Model file for the job. Use its own axes, mm. A direction names the side the tool comes from. Coordinates: 2 decimals unless noted, no trailing zeros. Order: outer loops, then holes, each group sorted by start corner. A loop starts at its lowest first (then second) coordinate and runs counter-clockwise, first axis right, second up. Notation, with made-up numbers: M 26.25,26 L 31.25,26 A29 ccw 31.25,60 Z; hole C -9.75,-25 d9. An arc over 180 degrees is marked long. Return JSON: item names as keys, results as strings.
```python
from build123d import *

# Parameters (mm, degrees)
BOSS_EXTRUDE1_DEPTH = 3
SKETCH2_R           = 1.5
CUT_EXTRUDE3_DEPTH  = 3
CUT_EXTRUDE4_START  = -10
CUT_EXTRUDE4_DEPTH  = 10
BOSS_EXTRUDE2_START = -3
BOSS_EXTRUDE2_DEPTH = 3
SKETCH5_W           = 0.56
SKETCH5_H           = 32.898596714
CUT_EXTRUDE5_DEPTH  = 3
SKETCH6_W           = 0.2
SKETCH6_H           = 32.898596714
CUT_EXTRUDE6_DEPTH  = 3
SKETCH7_R           = 2
CUT_EXTRUDE8_DEPTH  = 3
BOSS_EXTRUDE3_START = -3
BOSS_EXTRUDE3_DEPTH = 3
CUT_EXTRUDE9_START  = -3
CUT_EXTRUDE9_DEPTH  = 3
BOSS_EXTRUDE5_START = -3
BOSS_EXTRUDE5_DEPTH = 3
CUT_EXTRUDE10_START = -2
CUT_EXTRUDE10_DEPTH = 2
CUT_EXTRUDE11_START = -3
CUT_EXTRUDE11_DEPTH = 3
SKETCH13_R          = 1.5
CUT_EXTRUDE12_DEPTH = 1
SKETCH15_R          = 1.5
CUT_EXTRUDE13_DEPTH = 10


with BuildPart() as part:
    # Sketch1 → Boss-Extrude1 (new body)
    with BuildSketch(Plane.XY):
        with BuildLine():
            Line((-11, 25.5), (-22.790038711, 29.780264196))
            ThreePointArc((-22.790038711, 29.780264196), (0, -37.5), (22.790038711, 29.780264196))
            Line((22.790038711, 29.780264196), (11, 25.5))
            Line((11, 25.5), (-11, 25.5))
        make_face()
    extrude(amount=BOSS_EXTRUDE1_DEPTH)

    # Sketch2 → Cut-Extrude3 (cut)
    with BuildSketch(Plane.XY.offset(3)):
        with Locations((-25.400000001, 10.496905453)):
            Circle(SKETCH2_R)
        with Locations((-25.399981845, -10.493094547)):
            Circle(SKETCH2_R)
        with Locations(Location((25.399981845, -10.493094547, 0), (0, 0, 180))):
            Circle(SKETCH2_R)
        with Locations(Location((25.400000001, 10.496905453, 0), (0, 0, 180))):
            Circle(SKETCH2_R)
    extrude(amount=-CUT_EXTRUDE3_DEPTH, mode=Mode.SUBTRACT)

    # Sketch3 → Cut-Extrude4 (cut)
    with BuildSketch(Plane.XY.offset(3).offset(CUT_EXTRUDE4_START)):
        with BuildLine():
            Line((-30.76, 21.449298357), (-30.76, -21.449298357))
            ThreePointArc((-30.76, -21.449298357), (-37.5, 0), (-30.76, 21.449298357))
        make_face()
        with BuildLine():
            Line((30.76, 21.449298357), (30.76, -21.449298357))
            ThreePointArc((30.76, -21.449298357), (37.5, 0), (30.76, 21.449298357))
        make_face()
    extrude(amount=CUT_EXTRUDE4_DEPTH, mode=Mode.SUBTRACT)

    # Sketch4 → Boss-Extrude2 (add)
    with BuildSketch(Plane.XY.offset(3).offset(BOSS_EXTRUDE2_START)):
        with BuildLine():
            Line((-30.76, -21.449298357), (-30.76, -16.449298357))
            Line((-30.76, -16.449298357), (-33.699711921, -16.449298357))
            ThreePointArc((-33.699711921, -16.449298357), (-32.32667034, -19.006219634), (-30.76, -21.449298357))
        make_face()
        with BuildLine():
            Line((-33.699711921, 16.449298357), (-30.76, 16.449298357))
            Line((-30.76, 16.449298357), (-30.76, 21.449298357))
            ThreePointArc((-30.76, 21.449298357), (-32.32667034, 19.006219634), (-33.699711921, 16.449298357))
        make_face()
        with BuildLine():
            Line((30.76, 21.449298357), (30.76, 16.449298357))
            Line((30.76, 16.449298357), (33.699711921, 16.449298357))
            ThreePointArc((33.699711921, 16.449298357), (32.32667034, 19.006219634), (30.76, 21.449298357))
        make_face()
        with BuildLine():
            Line((30.76, -16.449298357), (30.76, -21.449298357))
            ThreePointArc((30.76, -21.449298357), (32.32667034, -19.006219634), (33.699711921, -16.449298357))
            Line((33.699711921, -16.449298357), (30.76, -16.449298357))
        make_face()
    extrude(amount=BOSS_EXTRUDE2_DEPTH)

    # Sketch5 → Cut-Extrude5 (cut)
    with BuildSketch(Plane.XY.offset(3)):
        with Locations((-30.48, 0)):
            Rectangle(SKETCH5_W, SKETCH5_H)
        with Locations((30.48, 0)):
            Rectangle(SKETCH5_W, SKETCH5_H)
    extrude(amount=-CUT_EXTRUDE5_DEPTH, mode=Mode.SUBTRACT)

    # Sketch6 → Cut-Extrude6 (cut)
    with BuildSketch(Plane.XY.offset(3)):
        with Locations((-30.1, 0)):
            Rectangle(SKETCH6_W, SKETCH6_H)
        with Locations((30.1, 0)):
            Rectangle(SKETCH6_W, SKETCH6_H)
    extrude(amount=-CUT_EXTRUDE6_DEPTH, mode=Mode.SUBTRACT)

    # Sketch7 → Cut-Extrude8 (cut)
    with BuildSketch(Plane.XY.offset(3)):
        with Locations((-19.15, -21.55)):
            Circle(SKETCH7_R)
        with Locations(Location((19.15, -21.55, 0), (0, 0, 180))):
            Circle(SKETCH7_R)
    extrude(amount=-CUT_EXTRUDE8_DEPTH, mode=Mode.SUBTRACT)

    # Sketch8 → Boss-Extrude3 (add)
    with BuildSketch(Plane.XY.offset(3).offset(BOSS_EXTRUDE3_START)):
        with BuildLine():
            Line((-33.699711921, 16.449298357), (-37.299711921, 16.449298357))
            ThreePointArc((-37.299711921, 16.449298357), (-32.744884003, 23.851322108), (-26.390038711, 29.780264196))
            Line((-26.390038711, 29.780264196), (-22.790038711, 29.780264196))
            ThreePointArc((-22.790038711, 29.780264196), (-29.020710607, 23.749702226), (-33.699711921, 16.449298357))
        make_face()
        with BuildLine():
            Line((33.699711921, 16.449298357), (37.299711921, 16.449298357))
            ThreePointArc((37.299711921, 16.449298357), (32.744884003, 23.851322108), (26.390038711, 29.780264196))
            Line((26.390038711, 29.780264196), (22.790038711, 29.780264196))
            ThreePointArc((22.790038711, 29.780264196), (29.020710607, 23.749702226), (33.699711921, 16.449298357))
        make_face()
    extrude(amount=BOSS_EXTRUDE3_DEPTH)

    # Sketch9 → Cut-Extrude9 (cut)
    with BuildSketch(Plane.XY.offset(3).offset(CUT_EXTRUDE9_START)):
        with BuildLine():
            Line((4.733920151, -37.2), (-4.733920151, -37.2))
            ThreePointArc((-4.733920151, -37.2), (0, -37.5), (4.733920151, -37.2))
        make_face()
    extrude(amount=CUT_EXTRUDE9_DEPTH, mode=Mode.SUBTRACT)

    # Sketch10 → Boss-Extrude5 (add)
    with BuildSketch(Plane.XY.offset(3).offset(BOSS_EXTRUDE5_START)):
        with BuildLine():
            ThreePointArc((-4.733920151, -37.2), (-21.838816892, -30.484685938), (-33.699711921, -16.449298357))
            Line((-33.699711921, -16.449298357), (-37.299711921, -16.449298357))
            ThreePointArc((-37.299711921, -16.449298357), (-23.43831182, -30.624902723), (-4.733920151, -37.2))
        make_face()
        with BuildLine():
            ThreePointArc((33.699711921, -16.449298357), (21.838816892, -30.484685938), (4.733920151, -37.2))
            ThreePointArc((4.733920151, -37.2), (23.43831182, -30.624902723), (37.299711921, -16.449298357))
            Line((37.299711921, -16.449298357), (33.699711921, -16.449298357))
        make_face()
        with BuildLine():
            Line((4.733920151, -37.2), (-4.733920151, -37.2))
            ThreePointArc((-4.733920151, -37.2), (0, -37.457659609), (4.733920151, -37.2))
        make_face()
    extrude(amount=BOSS_EXTRUDE5_DEPTH)

    # Sketch11 → Cut-Extrude10 (cut)
    with BuildSketch(Plane.XY.offset(3).offset(CUT_EXTRUDE10_START)):
        with BuildLine():
            Line((-30, 16.449298357), (-30, 13.449298357))
            Line((-30, 13.449298357), (30, 13.449298357))
            Line((30, 13.449298357), (30, 16.449298357))
            Line((30, 16.449298357), (37.299711921, 16.449298357))
            ThreePointArc((37.299711921, 16.449298357), (32.744884003, 23.851322108), (26.390038711, 29.780264196))
            Line((26.390038711, 29.780264196), (22.790038711, 29.780264196))
            Line((22.790038711, 29.780264196), (11, 25.5))
            Line((11, 25.5), (-11, 25.5))
            Line((-11, 25.5), (-22.790038711, 29.780264196))
            Line((-22.790038711, 29.780264196), (-26.390038711, 29.780264196))
            ThreePointArc((-26.390038711, 29.780264196), (-32.744884003, 23.851322108), (-37.299711921, 16.449298357))
            Line((-37.299711921, 16.449298357), (-30, 16.449298357))
        make_face()
    extrude(amount=CUT_EXTRUDE10_DEPTH, mode=Mode.SUBTRACT)

    # Sketch12 → Cut-Extrude11 (cut)
    with BuildSketch(Plane.XY.offset(3).offset(CUT_EXTRUDE11_START)):
        with BuildLine():
            Line((-30, 13.449298357), (-30, -16.449298357))
            Line((-30, -16.449298357), (-37.299711921, -16.449298357))
            ThreePointArc((-37.299711921, -16.449298357), (0, -37.457659609), (37.299711921, -16.449298357))
            Line((37.299711921, -16.449298357), (30, -16.449298357))
            Line((30, -16.449298357), (30, 13.449298357))
            Line((30, 13.449298357), (-30, 13.449298357))
        make_face()
    extrude(amount=CUT_EXTRUDE11_DEPTH, mode=Mode.SUBTRACT)

    # Sketch13 → Cut-Extrude12 (cut)
    with BuildSketch(Plane.XY.offset(1)):
        with Locations((-28.590038711, 23.780264196)):
            Circle(SKETCH13_R)
        with Locations(Location((28.590038711, 23.780264196, 0), (0, 0, 180))):
            Circle(SKETCH13_R)
    extrude(amount=-CUT_EXTRUDE12_DEPTH, mode=Mode.SUBTRACT)

    # Sketch15 → Cut-Extrude13 (cut)
    with BuildSketch(Plane(origin=(0, 0, 0), x_dir=(-1, 0, 0), z_dir=(0, 0, -1))):
        with Locations((-16, 20.5)):
            Circle(SKETCH15_R)
        with Locations((16, 20.5)):
            Circle(SKETCH15_R)
    extrude(amount=-CUT_EXTRUDE13_DEPTH, mode=Mode.SUBTRACT)


solid = part.part
```
Item 1: Drop a flat-ended pin along its axis: pin 1 Ø0.5 at (x, z) = (-34, 0.5) entering from -Y. Give the stop position or say it passes through.
Check result:
{"pin 1": "stops at y = 16.45"}
Item 2: Saw through at D-D (y = 19.75). Write the cut outline in (x, z), and give its area (3 significant figures).
Check result:
{"outline": "M -35.6,0 L -17.3,0 L -17.3,1 L -35.6,1 Z; M -14.7,0 L 14.7,0 L 14.7,1 L -14.7,1 Z; M 17.3,0 L 35.6,0 L 35.6,1 L 17.3,1 Z", "area": "66.0 mm2"}
Item 3: 3-axis set-ups, long thin cutter, end or side, ignore diameter. For faces 4 (the flat face through (-16.81, 27.61, 0.49)), 5 (the cylindrical face through (-32.82, 23.76, 0.49)): which of +Z, -Z, +X, -X, +Y, -Y reach the whole face in a straight line?
Check result:
{"face 4": "+Z, -Z, +Y", "face 5": "+Z, -Z, -X, +Y"}
Item 4: Pull direction Y, two halves, no side cores. Call faces 1 (the cylindrical face through (32.82, 23.76, 0.49)), 2 (the cylindrical face through (-30.09, 23.85, 0.51)), 3 (the flat face through (-1, 20, 1)): +Y half, -Y half, draft (parallel to the pull), parting line (faces both ways), or undercut.
Check result:
{"face 1": "+Y half", "face 2": "undercut", "face 3": "draft"}
Item 5: Saw through at A-A (y = 28.75). Write the cut outline in (x, z), and give its area (3 significant figures).
Check result:
{"outline": "M -27.77,0 L -19.95,0 L -19.95,1 L -27.77,1 Z; M 19.95,0 L 27.77,0 L 27.77,1 L 19.95,1 Z", "area": "15.6 mm2"}
Item 6: Saw through at B-B (x = 16). Write the cut outline in (y, z).
Check result:
{"outline": "M 13.45,0 L 19,0 L 19,1 L 13.45,1 Z; M 22,0 L 27.32,0 L 27.32,1 L 22,1 Z"}
Item 7: Wall check: line 1 (X direction, y = 25, z = 0.55); line 2 (X direction, y = 21, z = 0.7); line 3 (X direction, y = 16, z = 0.25). Give the ranges that are in metal, low to high.
Check result:
{"line 1": "x = -31.76 to -29.46, -27.72 to 27.72, 29.46 to 31.76", "line 2": "x = -34.83 to -17.41, -14.59 to 14.59, 17.41 to 34.83", "line 3": "x = -30 to 30"}
Item 8: Saw through at C-C (z = 0.5). Write the cut outline in (x, y).
Check result:
{"outline": "M -37.3,16.45 L -30,16.45 L -30,13.45 L 30,13.45 L 30,16.45 L 37.3,16.45 A32.48 ccw 26.39,29.78 L 22.79,29.78 L 11,25.5 L -11,25.5 L -22.79,29.78 L -26.39,29.78 A32.48 ccw Z; hole C -28.59,23.78 d3; hole C -16,20.5 d3; hole C 16,20.5 d3; hole C 28.59,23.78 d3"}
